from build123d import *

# Parameters (mm, degrees)
SKETCH1_R             = 30
SKETCH1_R_2           = 20
BOSS_EXTRUDE1_DEPTH   = 6.5
BOSS_EXTRUDE1_2_DEPTH = 6.5
SKETCH1_R_3           = 25
SKETCH1_R_4           = 15
BOSS_EXTRUDE1_3_DEPTH = 6.5
BOSS_EXTRUDE1_4_DEPTH = 6.5
BOSS_EXTRUDE1_5_DEPTH = 6.5
BOSS_EXTRUDE2_DEPTH   = 5


with BuildPart() as part:
    # Sketch1 → Boss-Extrude1 (new, symmetric)
    with BuildSketch(Plane.XY):
        with Locations(Location((0, 0, 0), (0, 0, 180))):
            Circle(SKETCH1_R)
        with Locations(Location((0, 0, 0), (0, 0, 180))):
            Circle(SKETCH1_R_2, mode=Mode.SUBTRACT)
    extrude(amount=BOSS_EXTRUDE1_DEPTH, both=True)



with BuildPart() as body_2:
    # Sketch1 → Boss-Extrude1 2 (new, symmetric)
    with BuildSketch(Plane.XY):
        with Locations(Location((-70, -98, 0), (0, 0, 180))):
            Circle(SKETCH1_R)
        with Locations(Location((-70, -98, 0), (0, 0, 180))):
            Circle(SKETCH1_R_2, mode=Mode.SUBTRACT)
    extrude(amount=BOSS_EXTRUDE1_2_DEPTH, both=True)


with BuildPart() as body_3:
    # Sketch1 → Boss-Extrude1 3 (new, symmetric)
    with BuildSketch(Plane.XY):
        with Locations(Location((-50, -185, 0), (0, 0, 180))):
            Circle(SKETCH1_R_3)
        with Locations(Location((-50, -185, 0), (0, 0, 180))):
            Circle(SKETCH1_R_4, mode=Mode.SUBTRACT)
    extrude(amount=BOSS_EXTRUDE1_3_DEPTH, both=True)


with BuildPart() as body_4:
    # Sketch1 → Boss-Extrude1 4 (new, symmetric)
    with BuildSketch(Plane.XY):
        with Locations(Location((70, -98, 0), (0, 0, 180))):
            Circle(SKETCH1_R)
        with Locations(Location((70, -98, 0), (0, 0, 180))):
            Circle(SKETCH1_R_2, mode=Mode.SUBTRACT)
    extrude(amount=BOSS_EXTRUDE1_4_DEPTH, both=True)


with BuildPart() as body_5:
    # Sketch1 → Boss-Extrude1 5 (new, symmetric)
    with BuildSketch(Plane.XY):
        with Locations(Location((50, -185, 0), (0, 0, 180))):
            Circle(SKETCH1_R_3)
        with Locations(Location((50, -185, 0), (0, 0, 180))):
            Circle(SKETCH1_R_4, mode=Mode.SUBTRACT)
    extrude(amount=BOSS_EXTRUDE1_5_DEPTH, both=True)


with BuildPart() as part_1:
    add(part.part)

    add(body_2.part)  # Boss-Extrude2 merges body 2

    add(body_3.part)  # Boss-Extrude2 merges body 3

    add(body_4.part)  # Boss-Extrude2 merges body 4

    add(body_5.part)  # Boss-Extrude2 merges body 5
    # Sketch1_3 → Boss-Extrude2 (add, symmetric)
    with BuildSketch(Plane.XY):
        with BuildLine():
            ThreePointArc((29.974824802, 1.228770963), (29.99370554, 0.614514416), (30, 0))
            ThreePointArc((30, 0), (-0.614514416, -29.99370554), (-29.974824802, 1.228770963))
            ThreePointArc((-29.974824802, 1.228770963), (-44.809013245, -41.993561968), (-80.883915711, -70.04395631))
            ThreePointArc((-80.883915711, -70.04395631), (-53.066563718, -73.235938627), (-40, -98))
            ThreePointArc((-40, -98), (-59.649329868, -126.157834217), (-92.857575187, -117.430163575))
            ThreePointArc((-92.857575187, -117.430163575), (-76.859583983, -147.370140698), (-74.716930719, -181.248555502))
            ThreePointArc((-74.716930719, -181.248555502), (-48.118945506, -160.070867765), (-25, -185))
            ThreePointArc((-25, -185), (-28.521882675, -197.794157893), (-38.095238095, -206.983553944))
            ThreePointArc((-38.095238095, -206.983553944), (0, -197.330926563), (38.095238095, -206.983553944))
            ThreePointArc((38.095238095, -206.983553944), (35.626049477, -164.54542725), (74.716930719, -181.248555502))
            ThreePointArc((74.716930719, -181.248555502), (76.859583983, -147.370140698), (92.857575187, -117.430163575))
            ThreePointArc((92.857575187, -117.430163575), (40.914175072, -105.349475372), (80.883915711, -70.04395631))
            ThreePointArc((80.883915711, -70.04395631), (44.809013245, -41.993561968), (29.974824802, 1.228770963))
        make_face()
    extrude(amount=BOSS_EXTRUDE2_DEPTH, both=True)


solid = part_1.part
The model under review builds one solid part; all positions refer to its coordinate system, in mm. A direction names the side the tool comes from. Round coordinates to 2 decimals unless told otherwise and drop trailing zeros. Loops run counter-clockwise (first coordinate to the right, second up) from the corner with the lowest first, then second, coordinate; pieces in that order, holes last. Notation, with made-up numbers: (31.5, -19.5) -> (71.5, -19.5) arc R28 cw to (71.5, 2.5) -> close; hole circle Ø10 at (89.5, -17). An arc over 180 degrees is marked (long way). Write item = value, one per line. Start each with the question number.
Item 1: Take a section at D-D on y = -17. Give the boundary of the cut face in (x, z).
Item 2: Take a section at C-C on z = -0.75. Give the boundary of the cut face in (x, y).
Item 3: Take a section at A-A on y = -185. Give the boundary of the cut face in (x, z), plus the area to 3 significant figures.
Item 4: To check wall thickness, follow L1, parallel to X at y = -185, z = -2; L2, parallel to Y at x = 62, z = 0.75; L3, parallel to Y at x = 52.5, z = 1.25. State the ranges of each line that lie inside material, in increasing order.
Item 5: Take a section at B-B on x = 0. Give the boundary of the cut face in (y, z).
Item 6: For faces 1 (the flat face through (50, -92, 6.5)), 2 (the cylindrical face through (-97.712, -86.51, 0.091)), 3 (the flat face through (-1, -101, 5)), list the 3-axis set-ups (+Z, -Z, +X, -X, +Y, -Y) from which the entire face can be reached by the end or side of a thin tool; tool diameter is ignored.
Item 7: Insertion check: pin 1 (1.5 mm diameter, centred on y = -19, z = -5, fed in from -X); pin 2 (6 mm diameter, centred on x = -51.5, z = -4, fed in from +Y); pin 3 (3 mm diameter, centred on y = 1.5, z = 1, fed in from +X). Each pin has a flat end and moves straight along its axis. Give the tip position at first contact, or say it passes through.
Result:
q1.outline = (-32.85, -5) -> (-24.72, -5) -> (-24.72, -6.5) -> (-10.54, -6.5) -> (-10.54, 6.5) -> (-24.72, 6.5) -> (-24.72, 5) -> (-32.85, 5) -> close; (10.54, -6.5) -> (24.72, -6.5) -> (24.72, -5) -> (32.85, -5) -> (32.85, 5) -> (24.72, 5) -> (24.72, 6.5) -> (10.54, 6.5) -> close
q2.outline = (-92.86, -117.43) arc R80 cw to (-74.72, -181.25) arc R25 ccw to (-38.1, -206.98) arc R80 cw to (38.1, -206.98) arc R25 ccw to (74.72, -181.25) arc R80 cw to (92.86, -117.43) arc R30 ccw to (80.88, -70.04) arc R80 cw to (29.97, 1.23) arc R30 ccw to (-29.97, 1.23) arc R80 cw to (-80.88, -70.04) arc R30 ccw to start; hole circle Ø40 at (-70, -98); hole circle Ø30 at (-50, -185); hole circle Ø40 at (0, 0); hole circle Ø30 at (50, -185); hole circle Ø40 at (70, -98)
q3.outline = (-75, -6.5) -> (-65, -6.5) -> (-65, 6.5) -> (-75, 6.5) -> close; (-35, -6.5) -> (-25, -6.5) -> (-25, -5) -> (25, -5) -> (25, -6.5) -> (35, -6.5) -> (35, 6.5) -> (25, 6.5) -> (25, 5) -> (-25, 5) -> (-25, 6.5) -> (-35, 6.5) -> close; (65, -6.5) -> (75, -6.5) -> (75, 6.5) -> (65, 6.5) -> close
q3.area = 1,020 mm²
q4.L1 = -75 to -65, -35 to 35, 65 to 75
q4.L2 = -206.93 to -194, -176 to -116.33, -79.67 to -59.56
q4.L3 = -209.87 to -199.79, -170.21 to -107.68, -88.32 to -51.21
q5.outline = (-197.33, -5) -> (-30, -5) -> (-30, -6.5) -> (-20, -6.5) -> (-20, 6.5) -> (-30, 6.5) -> (-30, 5) -> (-197.33, 5) -> close; (20, -6.5) -> (30, -6.5) -> (30, 6.5) -> (20, 6.5) -> close
q6.face_1 = +Z, +X, -X, +Y, -Y
q6.face_2 = none
q6.face_3 = +Z
q7.pin_1 = -33.67
q7.pin_2 = -46.77
q7.pin_3 = 30.03
